Autodesk Inventor part; units mm, degrees
ref_plane "YZ Plane" through (0, 0, 0) normal (1, 0, 0) x (0, 1, 0)
ref_plane "XZ Plane" through (0, 0, 0) normal (0, 1, 0) x (-1, 0, 0)
ref_plane "XY Plane" through (0, 0, 0) normal (0, 0, 1) x (1, 0, 0)
sketch "Sketch1" plane through (0, 0, 0) normal (0, 0, 1) x (1, 0, 0)
  point P0 (0, 0)
sketch "Sketch9" plane through (0, 0, 0) normal (0, 0, 1) x (1, 0, 0)
  line L0 (-12.03, 6.6772) -> (-12.03, 3.5022)
  line L1 (-13.62, 3.5022) -> (-13.62, 6.6772)
  line L2 (-12.05, 6.6772) -> (-13.62, 6.6772)
  line L3 (-13.62, 6.6772) -> (-12.03, 6.6772)
  line L4 (-13.62, 3.5022) -> (-12.03, 3.5022)
  point P0 (0, 0)
  dimension "d87" = 12.03
  dimension "d90" = 3.175
revolve "Revolution1" add sketch "Sketch9" angle 360 about axis through (-13.62, 3.5022, 0) along (1, 0, 0)
sketch "Sketch10" plane through (-12.03, 3.5022, 0) normal (1, 0, 0) x (0, 0, -1)
  circle A0 centre (0.0724, 0) radius 1.45
  point P0 (0, -3.5022)
fillet "Fillet11" radius 0.2 2 edges at (-12.03, 0.3272, 0) (-13.62, 0.3272, 0)
extrude "Extrusion7" add sketch "Sketch10" along normal blind 2.1
sketch "Sketch12" plane through (-9.93, 3.5022, -0.0724) normal (1, 0, 0) x (0, 0, -1)
  circle A0 centre (0, 0) radius 1.45
  circle A1 centre (0, 0) radius 0.5
  point P0 (-0.0724, -3.5022)
extrude "Extrusion10" cut sketch "Sketch12" against normal blind 0.1 contours A1
properties part number "falsarueda"
Check sheet for the modelled part. Datum: model origin and axes. Units: mm. Give positions to 0.01 mm unless a question says otherwise; leave off trailing zeros. Loops run counter-clockwise (first coordinate to the right, second up) from the corner with the lowest first, then second, coordinate; pieces in that order, holes last. Notation, with made-up numbers: M -21,57.25 L 15,57.25 A20 ccw 15,93.25 Z; hole C 1,7.5 d9. An arc over 180 degrees is marked long. Return JSON: item names as keys, results as strings. Group by question number.
1. Mould release check, pull along Y, two halves, no side actions. Record for faces 1 (the flat face through (-10.03, 3.5, -0.1)), 2 (the cylindrical face through (-10.99, 4.79, -0.74)), 3 (the flat face through (-12.03, 3, 2)): released by +Y, released by -Y, zero draft, split by the parting line, or undercut.
2. Thickness scan on L1, parallel to X at y = 4.5, z = 2; L2, parallel to Y at x = -10.15, z = 0; L3, parallel to Y at x = -13.3, z = 1.5. Record the ranges inside material, lowest first.
3. Cross-section at A-A on x = -12.4. Record the boundary of the cut face in (y, z) (3 decimals).
4. Cross-section at B-B on x = -10.7. Record the boundary of the cut face in (y, z), plus the area to 3 significant figures.
5. Go/stop test with a flat-tipped pin: pin 1 (1 mm diameter, centred on x = -12.5, z = -1, fed in from -Y). Record where the tip stops, or that it passes through.
Return value:
{
 "1": {"face 1": "undercut", "face 2": "split by the parting line", "face 3": "zero draft"},
 "2": {"L1": "-13.62 to -12.03", "L2": "2.05 to 4.95", "L3": "0.7 to 6.3"},
 "3": {"outline": "C 3.502,0 d6.35"},
 "4": {"outline": "C 3.5,-0.07 d2.9", "area": "6.61 mm^2"},
 "5": {"pin 1": "y = 0.37"}
}
